Can you work these out from the model? Positions are in its coordinate system, mm. A direction names the side the tool comes from. Coordinates: 2 decimals unless noted, no trailing zeros. Order: outer loops, then holes, each group sorted by start corner. A loop starts at its lowest first (then second) coordinate and runs counter-clockwise, first axis right, second up. Notation, with made-up numbers: (86.5, -37.5) -> (134.5, -37.5) arc R10 ccw to (134.5, -21.5) -> close; hole circle Ø1 at (-28, -24.75). An arc over 180 degrees is marked (long way). Return JSON: item names as keys, results as strings. Group by question number.
1) If I drill on probe 1 along X at (y, z) = (2.25, 0); probe 2 along Z at (x, y) = (20, 3.85); probe 3 along Y at (x, z) = (16.5, 12), over which ranges is the centre line in solid material (lowest first)? Write a range as from..to.
2) If we section it at C-C, the plane y = 40: Please give me the cut outline in (x, z), then the cut area to 3 significant figures.
3) If we section it at D-D, the plane z = 6: Please give me the cut outline in (x, y).
4) For pin 1 (20 mm diameter, centred on x = -2, y = 13, fed in from +Z) (3 decimals); pin 2 (10.5 mm diameter, centred on x = -20, z = 0, fed in from +Y); pin 3 (2 mm diameter, centred on x = -4.5, y = 11, fed in from +Z); pin 4 (5 mm diameter, centred on y = 40, z = 7.32, fed in from -X), each with a flat end and sliding along its axis, tell me the tip position at first contact or that it passes through.
5) If we section it at B-B, the plane z = -2.5: Please give me the cut outline in (x, y).
6) If we section it at A-A, the plane x = 20: Please give me the cut outline in (y, z), then the cut area to 3 significant figures.
7) For faces 5 (the cylindrical face through (-6.781, 33.034, -6.246)), 6 (the cylindrical face through (6.781, 26.617, 3.209)), 7 (the flat face through (-9, 16, 0)), 8 (the flat face through (30, 2, 0)), 9 (the flat face through (9, 16, 0)), which set-ups out of +Z, -Z, +X, -X, +Y, -Y let a thin tool reach every point of the face, with its end or its side?
8) Thinking about a two-plate mould opening in Z: for faces 1 (the cylindrical face through (-6.719, 26.704, 14.113)), 2 (the cylindrical face through (6.719, 33.034, -6.246)), 3 (the flat face through (17, 5, -4)), 4 (the flat face through (0, 10, 15)), which applies, +Z half, -Z half, draft (parallel to the pull), parting line (faces both ways), or undercut?
from build123d import *

# Parameters (mm, degrees)
SKETCH1_R           = 3.999999999999999
BOSS_EXTRUDE1_DEPTH = 5
SKETCH2_R           = 12.500000000000002
SKETCH2_R_2         = 4.000000000000002
BOSS_EXTRUDE2_DEPTH = 4.5
BOSS_EXTRUDE3_DEPTH = 9
FILLET1_R           = 2


with BuildPart() as part:
    # Sketch1 → Boss-Extrude1 (new body)
    with BuildSketch(Plane(origin=(0, 0, 0), x_dir=(1, 0, 0), z_dir=(0, 1, 0))):
        with BuildLine():
            Line((-21.999999999999943, -15), (21.999999999999943, -15))
            ThreePointArc((21.999999999999943, -15), (27.65685424949238, -12.65685424949238), (30, -6.999999999999942))
            Line((30, -6.999999999999942), (30, 6.999999999999942))
            ThreePointArc((30, 6.999999999999942), (27.65685424949238, 12.65685424949238), (21.999999999999943, 15))
            Line((21.999999999999943, 15), (-21.999999999999943, 15))
            ThreePointArc((-21.999999999999943, 15), (-27.656854249492383, 12.65685424949238), (-30.000000000000004, 6.999999999999942))
            Line((-30.000000000000004, 6.999999999999942), (-30.000000000000004, -6.999999999999942))
            ThreePointArc((-30.000000000000004, -6.999999999999942), (-27.656854249492383, -12.656854249492383), (-21.999999999999943, -15))
        make_face()
        with Locations(Location((-20.000000000000004, 0, 0), (0, 0, 270))):
            Circle(SKETCH1_R, mode=Mode.SUBTRACT)
        with Locations(Location((19.99999999999999, 0, 0), (0, 0, 90))):
            Circle(SKETCH1_R, mode=Mode.SUBTRACT)
    extrude(amount=BOSS_EXTRUDE1_DEPTH)

    # Sketch2 → Boss-Extrude2 (add, symmetric)
    # profile 1 of 3: a face of its own
    with BuildSketch(Plane(origin=(0, 0, 0), x_dir=(0, 0, -1), z_dir=(1, 0, 0))):
        with BuildLine():
            ThreePointArc((-15, 28.295090269147053), (-1.9659638137879094, 27.06388231319019), (6.386690828752239, 37.145307448395535))
            Line((6.386690828752239, 37.145307448395535), (15.000000000000002, 5))
            Line((15.000000000000002, 5), (-15, 5))
            Line((-15, 5), (-15, 28.295090269147053))
        make_face()
    # profile 2 of 3: a face of its own
    with BuildSketch(Plane(origin=(0, 0, 0), x_dir=(0, 0, -1), z_dir=(1, 0, 0))):
        with BuildLine():
            Line((-19.39324681882872, 36.76476193621847), (-15, 20.368941598159466))
            Line((-15, 20.368941598159466), (-15, 28.295090269147053))
            ThreePointArc((-15, 28.295090269147053), (-1.9659638137879103, 27.06388231319019), (6.386690828752242, 37.145307448395535))
            Line((6.386690828752239, 37.145307448395535), (4.754898838397972, 43.23523806378153))
            ThreePointArc((4.754898838397979, 43.23523806378153), (5.073886776957259, 41.63157740275066), (5.1808260097846315, 40))
            ThreePointArc((5.1808260097846315, 40), (-5.687596587464719, 27.60693923282737), (-19.39324681882872, 36.76476193621848))
        make_face()
    # profile 3 of 3: a face of its own
    with BuildSketch(Plane(origin=(0, 0, 0), x_dir=(0, 0, -1), z_dir=(1, 0, 0))):
        with Locations((-7.31917399021537, 40)):
            Circle(SKETCH2_R)
        with Locations((-7.31917399021537, 40)):
            Circle(SKETCH2_R_2, mode=Mode.SUBTRACT)
    extrude(amount=BOSS_EXTRUDE2_DEPTH, both=True)

    # Sketch2_4 → Boss-Extrude3 (add, symmetric)
    with BuildSketch(Plane(origin=(0, 0, 0), x_dir=(0, 0, -1), z_dir=(1, 0, 0))):
        with BuildLine():
            ThreePointArc((-15, 28.295090269147053), (-1.9659638137879094, 27.06388231319019), (6.386690828752239, 37.145307448395535))
            Line((6.386690828752239, 37.145307448395535), (15.000000000000002, 5))
            Line((15.000000000000002, 5), (-15, 5))
            Line((-15, 5), (-15, 28.295090269147053))
        make_face()
    extrude(amount=BOSS_EXTRUDE3_DEPTH, both=True)

    # Fillet1
    fillet1_edges = [part.edges().sort_by_distance(p)[0] for p in [
        (-6.75, 37.145307448395535, -6.38669082875224),
        (-6.75, 28.295090269147053, 15),
        (6.75, 37.145307448395535, -6.38669082875224),
        (6.75, 28.295090269147053, 15),
    ]]
    fillet(fillet1_edges, radius=FILLET1_R)


solid = part.part
Result sheet:
{
 "1": {"probe 1": "x = -30..-24, -16..16, 24..30", "probe 2": "z = -15..-4, 4..15", "probe 3": "y = 0..5"},
 "2": {"outline": "(-4.5, -5.62) -> (4.5, -5.62) -> (4.5, 3.32) -> (-4.5, 3.32) -> close; (-4.5, 11.32) -> (4.5, 11.32) -> (4.5, 19.82) -> (-4.5, 19.82) -> close", "area": "157 mm2"},
 "3": {"outline": "(-30, 0) -> (30, 0) -> (30, 5) -> (9, 5) -> (9, 26.06) -> (4.5, 26.06) -> (4.5, 36.22) -> (-4.5, 36.22) -> (-4.5, 26.06) -> (-9, 26.06) -> (-9, 5) -> (-30, 5) -> close; (-4.5, 43.78) -> (4.5, 43.78) -> (4.5, 52.43) -> (-4.5, 52.43) -> close"},
 "4": {"pin 1": "stops at z = 15.705", "pin 2": "stops at y = 5", "pin 3": "stops at z = 15", "pin 4": "passes through"},
 "5": {"outline": "(-30, 0) -> (-23.12, 0) -> (-23.12, 5) -> (-30, 5) -> close; (-16.88, 0) -> (16.88, 0) -> (16.88, 5) -> (9, 5) -> (9, 30.02) -> (4.5, 30.02) -> (4.5, 47.74) -> (-4.5, 47.74) -> (-4.5, 30.02) -> (-9, 30.02) -> (-9, 5) -> (-16.88, 5) -> close; (23.12, 0) -> (30, 0) -> (30, 5) -> (23.12, 5) -> close"},
 "6": {"outline": "(0, -15) -> (5, -15) -> (5, -4) -> (0, -4) -> close; (0, 4) -> (5, 4) -> (5, 15) -> (0, 15) -> close", "area": "110 mm2"},
 "7": {"face 5": "-X, +Y", "face 6": "+X, +Y", "face 7": "+Z, -Z, -X, +Y", "face 8": "+Z, -Z, +X, +Y, -Y", "face 9": "+Z, -Z, +X, +Y"},
 "8": {"face 1": "undercut", "face 2": "parting line", "face 3": "draft", "face 4": "+Z half"}
}
